For this review, take the finished solid that the model builds, in its own axes (mm). A direction names the side the tool comes from. Coordinates: 2 decimals unless noted, no trailing zeros.
1. Mouldability with a two-part tool opening along Z and no side actions: class faces 4 (the face through (17.68, -2.96, -4.36)), 5 (the face through (18, -6, -1)), 6 (the face through (18, -13, 26)), 7 (the face through (-10.916, -18.686, -14.522)) as pulls with the +Z half, pulls with the -Z half, needs draft (parallel to the pull), parting line crosses it, or undercut.
2. Machinability: for faces 1 (the face through (-0.1, -23.6, -26)), 2 (the face through (-17, -6, 3)), 3 (the face through (16.302, -16.353, 9.731)), which of the approach directions +Z, -Z, +X, -X, +Y, -Y give a long, thin tool a straight path to every point of the face, cutting with its end or side? Answer none if there is none.
3. To check wall thickness, follow probe 1 along X at (y, z) = (-3.9, -4.8); probe 2 along X at (y, z) = (-4.2, -4.8); probe 3 along Z at (x, y) = (-2, -22). State the ranges of each line that lie inside material, in increasing order.
4. Clearance check with flat-ended pins moving along their axes: P1, Ø10, axis at y = -18.5, z = -2.5, coming from the +X side; P2, Ø10, axis at y = -11.5, z = 8, coming from the -X side; P3, Ø12, axis at x = -2, y = -8, coming from the +Z side; P4, Ø1.7, axis at x = -16.3, z = -4.8, coming from the +Y side. State where each tip first meets the part, or that it passes through.
5. Take a section at A-A, the plane y = -2.5. Count the separate pieces of the cut face and the enclosed holes in it, then the cut area to 3 significant figures.
```python
from build123d import *

# Parameters (mm, degrees)
F0_R          = 1.45
F1_DEPTH      = 27
F3_START      = 6
F3_DEPTH      = 23
F6_W          = 32
F6_H          = 11.5
F9_DEPTH      = 25
F9_DEPTH_BACK = 25
F6_W_2        = 27
F6_H_2        = 18


with BuildPart() as f1:
    # F0 (on Front) → F1 (new body)
    with BuildSketch(Plane.XZ):
        Polygon((-8.5, -26), (8.5, -26), (20, -10), (20, 26), (-20, 26), (-20, -10), align=None)
        with Locations((-16.3, -4.8)):
            Circle(F0_R, mode=Mode.SUBTRACT)
        with Locations((16.3, -4.8)):
            Circle(F0_R, mode=Mode.SUBTRACT)
    extrude(amount=F1_DEPTH)

    # F2 (on Front) → F3 (cut)
    with BuildSketch(Plane.XZ.offset(F3_START)):
        Polygon((26.5, -25), (26.499954751, 0.0001809961), (20, 26), (12.5, -7), (8.5, -26), align=None)
        Polygon((-8.5, -26), (-12.5, -7), (-20, 26), (-26.499954751, 0.0001809961), (-26.5, -25), align=None)
    extrude(amount=F3_DEPTH, mode=Mode.SUBTRACT)

    # F6 (on Front) → F7 section 0
    with BuildSketch(Plane.XZ):
        with Locations((0, 20.25)):
            Rectangle(F6_W, F6_H)
    # F5 (on offset) → F7 section 1
    with BuildSketch(Plane.XZ.offset(27)):
        Polygon((8, -11), (16, 26), (-16, 26), (-8, -11), align=None)
    loft(mode=Mode.SUBTRACT)

    # F8 (on Right) → F9 (cut, two sides)
    with BuildSketch(Plane.YZ) as f9_sk:
        Polygon((-5.9656337835, -11.392949149), (-27.1901637316, -30.3732156754), (3.7769323681, -39.4357405603), (2.9211663641, -11.3271204755), align=None)
    extrude(amount=-F9_DEPTH, mode=Mode.SUBTRACT)
    extrude(f9_sk.sketch, amount=F9_DEPTH_BACK, mode=Mode.SUBTRACT)

    # F6 (on Front) → F10 section 0
    with BuildSketch(Plane.XZ):
        with Locations((0, 3)):
            Rectangle(F6_W_2, F6_H_2)
    # F5 (on offset) → F10 section 1
    with BuildSketch(Plane.XZ.offset(27)):
        Polygon((5.5, -28.406675905), (6.5, -14), (-6.5, -14), (-5.5, -28.406675905), align=None)
    loft(mode=Mode.SUBTRACT)


solid = f1.part
```
Results list:
1. face 4: undercut
1. face 5: needs draft
1. face 6: pulls with the +Z half
1. face 7: pulls with the -Z half
2. face 1: -Z, +X, -X, +Y, -Y
2. face 2: -Z, -X, -Y
2. face 3: -Z, +X, -Y
3. probe 1: x = -20 to -17.75, -14.85 to -12.38, 12.38 to 14.85, 17.75 to 20
3. probe 2: x = -20 to -17.75, -14.85 to -12.3, 12.3 to 14.85, 17.75 to 20
3. probe 3: z = -25.73 to -24.26, -9.19 to -6.28
4. P1: stops at x = 14.66
4. P2: stops at x = -17.05
4. P3: stops at z = 12.61
4. P4: passes through
5. separate pieces: 1
5. enclosed holes: 3
5. area: 594 mm2
